Check sheet for the modelled part. Datum: model origin and axes. Units: mm. A direction names the side the tool comes from. Give positions to 0.01 mm unless a question says otherwise; leave off trailing zeros. Write each loop counter-clockwise with the first axis right and the second up, starting at its lowest first coordinate (ties: lowest second). Pieces come first, ordered by that corner, then holes. Notation, with made-up numbers: M 44.5,73 L 82.5,73 A20 cw 82.5,91 Z; hole C 41.25,44 d4. An arc over 180 degrees is marked long. Write item = value, one per line. Start each with the question number.
1) Cross-section at C-C, the plane y = -185. Record the cut outline in (x, z), plus the area to 3 significant figures.
2) Cross-section at B-B, the plane z = 0. Record the cut outline in (x, y).
3) Mould release check, pull along Z, two halves, no side actions. Record for faces 1 (the flat face through (-6.26, -83.81, 11.05)), 2 (the cylindrical face through (1.08, 14.79, -4.88)), 3 (the flat face through (0, 30, 0)): released by +Z, released by -Z, zero draft, split by the parting line, or undercut.
4) Cross-section at D-D, the plane z = 9.25. Record the cut outline in (x, y), plus the area to 3 significant figures.
5) Go/stop test with flat-tipped pins: pin 1 (8 mm diameter, centred on y = -66.5, z = -11.5, fed in from +X); pin 2 (2 mm diameter, centred on x = 10, y = -68.5, fed in from -Z). Record where each tip stops, or that it passes through.
6) Scan lines: line 1 along Y through (x, z) = (-3.5, -12); line 2 along Z through (x, y) = (8.25, -161); line 3 along X through (y, z) = (-64, 12.5). Record each from-to range of solid material in increasing order. Write a range as [from, to].
7) Access from +Z, -Z, +X, -X, +Y, -Y to the whole of each face (thin tool, end or side, straight path). Record for faces 4 (the flat face through (0, -170, -6)), 5 (the flat face through (0, 0, -6)), 6 (the flat face through (0, -200, 0)).
8) Cross-section at A-A, the plane y = -101. Record the cut outline in (x, z).
```python
from build123d import *

# Parameters (mm, degrees)
F1_DEPTH = 170
F2_R     = 5
F3_DEPTH = 30
F4_R     = 5
F5_DEPTH = 30


# Not quite as in the source:
# - a feature names something its author has since deleted; it is built from what else it names


with BuildPart() as f1:
    # F0 (on Front) → F1 (new body)
    with BuildSketch(Plane.XZ):
        Polygon((-12.7, 7.3323484187), (-12.7, -7.3323484187), (0, -14.6646968374), (12.7, -7.3323484187), (12.7, 7.3323484187), (0, 14.6646968374), align=None)
    extrude(amount=F1_DEPTH)

    # F2 (on face) → F3 (join)
    with BuildSketch(Plane(origin=(0, 0, 0), x_dir=(-1, 0, 0), z_dir=(0, 1, 0))):
        Circle(F2_R)
    extrude(amount=F3_DEPTH)

    # F4 (on face) → F5 (join)
    with BuildSketch(Plane.XZ.offset(170)):
        Circle(F4_R)
    extrude(amount=F5_DEPTH)


solid = f1.part
```
Reply:
q1.outline = C 0,0 d10
q1.area = 78.5 mm2
q2.outline = M -12.7,-170 L -5,-170 L -5,-200 L 5,-200 L 5,-170 L 12.7,-170 L 12.7,0 L 5,0 L 5,30 L -5,30 L -5,0 L -12.7,0 Z
q3.face_1 = released by +Z
q3.face_2 = split by the parting line
q3.face_3 = zero draft
q4.outline = M -9.38,-170 L 9.38,-170 L 9.38,0 L -9.38,0 Z
q4.area = 3,190 mm2
q5.pin_1 = 12.41
q5.pin_2 = -9.47
q6.line_1 = [-170, 0]
q6.line_2 = [-9.9, 9.9]
q6.line_3 = [-3.75, 3.75]
q7.face_4 = -Y
q7.face_5 = +Y
q7.face_6 = +Z, -Z, +X, -X, -Y
q8.outline = M -12.7,-7.33 L 0,-14.66 L 12.7,-7.33 L 12.7,7.33 L 0,14.66 L -12.7,7.33 Z
